```python
from build123d import *

# Parameters (mm, degrees)
SKETCH_1_W          = 72
SKETCH_1_H          = 14.5
EXTRUDE_1_DEPTH     = 3
SKETCH_2_W          = 72
SKETCH_2_H          = 3
EXTRUDE_2_DEPTH     = 80
SKETCH_3_W          = 3
SKETCH_3_H          = 13
EXTRUDE_3_DEPTH     = 13.5
SKETCH_4_R          = 2.5
CUT_EXTRUDE_1_DEPTH = 21
SKETCH_5_W          = 20
SKETCH_5_H          = 3
CUT_EXTRUDE_2_DEPTH = 21
SKETCH_6_W          = 3
SKETCH_6_H          = 14.5
EXTRUDE_5_DEPTH     = 2
SKETCH_8_W          = 3
SKETCH_8_H          = 80.708275322
EXTRUDE_6_DEPTH     = 18
CUT_EXTRUDE_3_DEPTH = 21
SKETCH_12_R         = 25
CUT_EXTRUDE_5_DEPTH = 8
CUT_EXTRUDE_6_DEPTH = 31


with BuildPart() as part:
    # 草图1 → 凸台-拉伸1 (new body)
    with BuildSketch(Plane.XY):
        with Locations((36, 7.25)):
            Rectangle(SKETCH_1_W, SKETCH_1_H)
    extrude(amount=EXTRUDE_1_DEPTH)

    # 草图2 → 凸台-拉伸2 (add)
    with BuildSketch(Plane.XY.offset(3)):
        with Locations((36, 1.5)):
            Rectangle(SKETCH_2_W, SKETCH_2_H)
        with Locations((36, 13)):
            Rectangle(SKETCH_2_W, SKETCH_2_H)
    extrude(amount=EXTRUDE_2_DEPTH)

    # 草图3 → 凸台-拉伸3 (add)
    with BuildSketch(Plane(origin=(0, 0, 0), x_dir=(-1, 0, 0), z_dir=(0, 0, -1))):
        with Locations((-39, 7.25)):
            Rectangle(SKETCH_3_W, SKETCH_3_H)
        Polygon((-43.5, 0.75), (-43.5, 7.25), (-43.5, 13.75), (-46.5, 13.75), (-46.5, 0.75), align=None)
        with Locations((-33, 7.25)):
            Rectangle(SKETCH_3_W, SKETCH_3_H)
        Polygon((-28.5, 7.25), (-28.5, 13.75), (-25.5, 13.75), (-25.5, 0.75), (-28.5, 0.75), align=None)
    extrude(amount=EXTRUDE_3_DEPTH)

    # 草图4 → 切除-拉伸1 (cut)
    with BuildSketch(Plane.ZY.offset(-25.5)):
        with Locations((-7, 7.25)):
            Circle(SKETCH_4_R)
        with BuildLine():
            Line((-7, 0.75), (-7, -0.932690229))
            Line((-7, -0.932690229), (-15.150689601, -0.932690229))
            Line((-15.150689601, -0.932690229), (-15.150689601, 14.849085894))
            Line((-15.150689601, 14.849085894), (-7, 13.75))
            ThreePointArc((-7, 13.75), (-13.5, 7.25), (-7, 0.75))
        make_face()
    extrude(amount=-CUT_EXTRUDE_1_DEPTH, mode=Mode.SUBTRACT)

    # 草图5 → 切除-拉伸2 (cut)
    with BuildSketch(Plane(origin=(0, 14.5, 0), x_dir=(1, 0, 0), z_dir=(0, 1, 0))):
        with Locations((13, -79.5)):
            Rectangle(SKETCH_5_W, SKETCH_5_H)
        with Locations((59, -79.5)):
            Rectangle(SKETCH_5_W, SKETCH_5_H)
    extrude(amount=-CUT_EXTRUDE_2_DEPTH, mode=Mode.SUBTRACT)

    # 草图6 → 凸台-拉伸5 (add)
    with BuildSketch(Plane(origin=(0, 0, 0), x_dir=(-1, 0, 0), z_dir=(0, 0, -1))):
        with Locations((-70.5, 7.25)):
            Rectangle(SKETCH_6_W, SKETCH_6_H)
        with Locations((-1.5, 7.25)):
            Rectangle(SKETCH_6_W, SKETCH_6_H)
    extrude(amount=EXTRUDE_5_DEPTH)

    # 草图8 → 凸台-拉伸6 (add)
    with BuildSketch(Plane(origin=(0, 13.75, 0), x_dir=(1, 0, 0), z_dir=(0, 1, 0))):
        with Locations((27, -33.354137661)):
            Rectangle(SKETCH_8_W, SKETCH_8_H)
        with Locations((33, -33.354137661)):
            Rectangle(SKETCH_8_W, SKETCH_8_H)
        with Locations((39, -33.354137661)):
            Rectangle(SKETCH_8_W, SKETCH_8_H)
        with Locations((45, -33.354137661)):
            Rectangle(SKETCH_8_W, SKETCH_8_H)
    extrude(amount=EXTRUDE_6_DEPTH)

    # 草图9 → 切除-拉伸3 (cut)
    with BuildSketch(Plane.ZY.offset(-25.5)):
        Polygon((-7, 31.75), (73.708275322, 14.5), (73.708275322, 31.75), align=None)
    extrude(amount=-CUT_EXTRUDE_3_DEPTH, mode=Mode.SUBTRACT)

    # 草图12 → 切除-拉伸5 (cut)
    with BuildSketch(Plane.XZ):
        with Locations((82, 36)):
            Circle(SKETCH_12_R)
    extrude(amount=-CUT_EXTRUDE_5_DEPTH, mode=Mode.SUBTRACT)

    # 草图13 → 切除-拉伸6 (cut)
    with BuildSketch(Plane.ZY.offset(-25.5)):
        Polygon((-7, 19.685447093), (-2.115986675, 30.7061265), (-3.141307931, 37.349064324), (-11.498288127, 31.75), align=None)
    extrude(amount=-CUT_EXTRUDE_6_DEPTH, mode=Mode.SUBTRACT)


solid = part.part
```
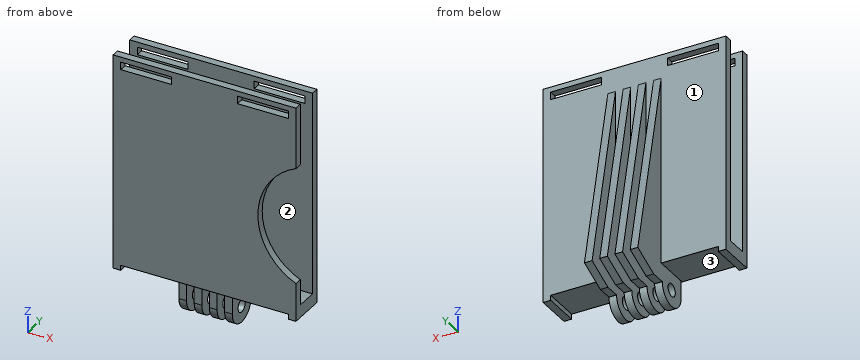
Input: part model. Units: mm. Frame: model coordinates. Face numbers are marked on the shaded views. Coordinates: 2 decimals unless noted, no trailing zeros. Loops run counter-clockwise (first coordinate to the right, second up) from the corner with the lowest first, then second, coordinate; pieces in that order, holes last. Notation, with made-up numbers: M 68,18 L 77,18 A33 cw 77,53 Z; hole C 17.25,51.25 d6. An arc over 180 degrees is marked long. Use a Markdown table: item, result. Add a question column.
1) Section B-B, the plane z = 56.5. Return the cut outline in (x, y).
2) Pin query (flat end, axial travel): P1, Ø1, axis at x = 56, z = 18.5, coming from the +Y side; P2, Ø2, axis at x = 41, z = 73, coming from the +Y side; P3, Ø5, axis at x = 26, z = 41.5, coming from the +Y side. Return the tip coordinate at first contact, or that it passes through.
3) Section D-D, the plane x = 65. Return the cut outline in (y, z), plus the area to 3 significant figures.
4) Section A-A, the plane x = 53.5. Return the cut outline in (y, z), plus the area to 4 significant figures.
5) Line query: L1, parallel to X at y = 16.5, z = 13; L2, parallel to Z at x = 50, y = 2.5; L3, parallel to Z at x = 38, y = 7. Output: solid intervals per line, ascending. Write a range as from..to.
6) Draft query along X for the marked faces 1, 2 and 3. Return one class per face: +X half, -X half, draft (parallel to the pull), parting line (faces both ways), or undercut.
7) Section C-C, the plane y = 23. Return the cut outline in (x, z), plus the area to 3 significant figures.
Answer below:
| question | item | result |
|---|---|---|
| 1 | outline | M 0,0 L 67.69,0 L 67.69,3 L 0,3 Z; M 0,11.5 L 72,11.5 L 72,14.5 L 46.5,14.5 L 46.5,18.18 L 43.5,18.18 L 43.5,14.5 L 40.5,14.5 L 40.5,18.18 L 37.5,18.18 L 37.5,14.5 L 34.5,14.5 L 34.5,18.18 L 31.5,18.18 L 31.5,14.5 L 28.5,14.5 L 28.5,18.18 L 25.5,18.18 L 25.5,14.5 L 0,14.5 Z |
| 2 | P1 | y = 14.5 |
| 2 | P2 | y = 14.84 |
| 2 | P3 | y = 21.92 |
| 3 | outline | M 0,0 L 14.5,0 L 14.5,78 L 11.5,78 L 11.5,3 L 3,3 L 3,17.67 L 0,17.67 Z; M 0,54.33 L 3,54.33 L 3,78 L 0,78 Z; M 0,81 L 3,81 L 3,83 L 0,83 Z; M 11.5,81 L 14.5,81 L 14.5,83 L 11.5,83 Z |
| 3 | area | 396 mm2 |
| 4 | outline | M 0,0 L 14.5,0 L 14.5,78 L 11.5,78 L 11.5,3 L 3,3 L 3,78 L 0,78 Z; M 0,81 L 3,81 L 3,83 L 0,83 Z; M 11.5,81 L 14.5,81 L 14.5,83 L 11.5,83 Z |
| 4 | area | 505.5 mm2 |
| 5 | L1 | 25.5..28.5, 31.5..34.5, 37.5..40.5, 43.5..46.5 |
| 5 | L2 | 0..78, 81..83 |
| 5 | L3 | -13.5..-9.49, -4.51..3 |
| 6 | face 1 | undercut |
| 6 | face 2 | draft |
| 6 | face 3 | undercut |
| 7 | outline | M 25.5,-5.53 L 28.5,-5.53 L 28.5,33.94 L 25.5,33.94 Z; M 31.5,-5.53 L 34.5,-5.53 L 34.5,33.94 L 31.5,33.94 Z; M 37.5,-5.53 L 40.5,-5.53 L 40.5,33.94 L 37.5,33.94 Z; M 43.5,-5.53 L 46.5,-5.53 L 46.5,33.94 L 43.5,33.94 Z |
| 7 | area | 474 mm2 |
